Part model, mm, in its own coordinate system. A direction names the side the tool comes from. Give positions to 0.01 mm unless a question says otherwise; leave off trailing zeros. Loops run counter-clockwise (first coordinate to the right, second up) from the corner with the lowest first, then second, coordinate; pieces in that order, holes last. Notation, with made-up numbers: M 70.25,-33 L 76.25,-33 A14 cw 76.25,-22 Z; hole C -15.5,37 d7. An arc over 180 degrees is marked long. Put each result on its own line as item: value. Start each with the question number.
```python
from build123d import *

# Parameters (mm, degrees)
BOSS_EXTRUDE1_DEPTH = 3
SKETCH2_W           = 5
SKETCH2_H           = 5
BOSS_EXTRUDE2_DEPTH = 3
SKETCH3_W           = 5
SKETCH3_H           = 5
BOSS_EXTRUDE4_DEPTH = 3
SKETCH4_R           = 1.5
CUT_EXTRUDE1_DEPTH  = 27.537709019
CHAMFER1_SIZE       = 7
CHAMFER1_SIZE2      = 4.901452767
CHAMFER2_SIZE       = 7
CHAMFER2_SIZE2      = 4.901452767
SKETCH6_W           = 11
SKETCH6_H           = 3.5
BOSS_EXTRUDE5_DEPTH = 4.5
SKETCH9_W           = 11
SKETCH9_H           = 3.5
BOSS_EXTRUDE6_DEPTH = 3
FILLET1_R           = 5.5
FILLET2_R           = 3
SKETCH16_R          = 1.5
CUT_EXTRUDE7_DEPTH  = 30.857997254
SKETCH17_R          = 3.05
CUT_EXTRUDE8_DEPTH  = 2
SKETCH18_W          = 3
SKETCH18_H          = 8
BOSS_EXTRUDE7_DEPTH = 1
SKETCH19_W          = 3
SKETCH19_H          = 8
BOSS_EXTRUDE8_DEPTH = 1


# Some blends are built 0.0001 mm under size
with BuildPart() as part:
    # Sketch1 → Boss-Extrude1 (new body)
    with BuildSketch(Plane(origin=(0, 0, 0), x_dir=(1, 0, 0), z_dir=(0, 1, 0))):
        Polygon((-7.5, -12.5), (-7.5, 2.962729178), (0, 8.214285714), (7.5, 2.962729178), (7.5, -12.5), (12.5, -12.5), (12.5, 12.5), (-12.5, 12.5), (-12.5, -12.5), align=None)
    extrude(amount=BOSS_EXTRUDE1_DEPTH)

    # Sketch2 → Boss-Extrude2 (add)
    with BuildSketch(Plane.XY.offset(12.5)):
        with Locations((-10, 5.5)):
            Rectangle(SKETCH2_W, SKETCH2_H)
    extrude(amount=-BOSS_EXTRUDE2_DEPTH)

    # Sketch3 → Boss-Extrude4 (add)
    with BuildSketch(Plane.XY.offset(12.5)):
        with Locations((10, 5.5)):
            Rectangle(SKETCH3_W, SKETCH3_H)
    extrude(amount=-BOSS_EXTRUDE4_DEPTH)

    # Sketch4 → Cut-Extrude1 (cut, through all)
    with BuildSketch(Plane(origin=(0, 0, 9.5), x_dir=(-1, 0, 0), z_dir=(0, 0, -1))):
        with Locations((10, 5.5)):
            Circle(SKETCH4_R)
        with Locations(Location((-10, 5.5, 0), (0, 0, 180))):
            Circle(SKETCH4_R)
    extrude(amount=-CUT_EXTRUDE1_DEPTH, mode=Mode.SUBTRACT)

    # Chamfer1
    chamfer1_edges = [part.edges().sort_by_distance(p)[0] for p in [
        (-12.5, 1.5, -12.5),
    ]]
    chamfer1_side = [part.faces().sort_by_distance(p)[0] for p in [
        (0, 1.5, -12.5),
    ]]
    chamfer(chamfer1_edges, length=CHAMFER1_SIZE, length2=CHAMFER1_SIZE2, reference=chamfer1_side[0])

    # Chamfer2
    chamfer2_edges = [part.edges().sort_by_distance(p)[0] for p in [
        (12.5, 1.5, -12.5),
    ]]
    chamfer2_side = [part.faces().sort_by_distance(p)[0] for p in [
        (3.5, 1.5, -12.5),
    ]]
    chamfer(chamfer2_edges, length=CHAMFER2_SIZE, length2=CHAMFER2_SIZE2, reference=chamfer2_side[0])

    # Sketch6 → Boss-Extrude5 (add)
    with BuildSketch(Plane(origin=(0, 3, 0), x_dir=(1, 0, 0), z_dir=(0, 1, 0))):
        with Locations((0, 10.75)):
            Rectangle(SKETCH6_W, SKETCH6_H)
    extrude(amount=BOSS_EXTRUDE5_DEPTH)

    # Sketch9 → Boss-Extrude6 (add)
    with BuildSketch(Plane(origin=(0, 7.5, 0), x_dir=(1, 0, 0), z_dir=(0, 1, 0))):
        with Locations((0, 10.75)):
            Rectangle(SKETCH9_W, SKETCH9_H)
    extrude(amount=BOSS_EXTRUDE6_DEPTH)

    # Fillet1
    fillet1_edges = [part.edges().sort_by_distance(p)[0] for p in [
        (5.5, 10.5, -10.75),
        (-5.5, 10.5, -10.75),
    ]]
    fillet(fillet1_edges, radius=FILLET1_R - 0.0001)  # a hair under: the kernel refuses the full size

    # Fillet2
    # the kernel refuses this fillet: 3 mm, written as the material it adds along each edge
    with BuildSketch(Plane(origin=(-5.5, 3, -9), x_dir=(-1, 0, 0), z_dir=(0, 0, -1))) as fillet2_piece_1_section:
        with BuildLine():
            CenterArc((2.940982655, 3), FILLET2_R, 186.755728099, 83.244271901)
            Line((-0.038187449, 2.647089966), (-0.336104459, 2.611798962))
            ThreePointArc((-0.336104459, 2.611798962), (-0.3, 2.0001), (-0.3, 0))
            Line((-0.3, 0), (0, -0.3))
            Line((0, -0.3), (2.940982655, -0.3))
            Line((2.940982655, -0.3), (2.940982655, 0))
        make_face()
    fillet2_piece_1 = extrude(amount=3.5, mode=Mode.PRIVATE)
    fillet2_piece_1 = split(fillet2_piece_1, bisect_by=Plane(origin=(-8.304245999, 3.032166693, -10.536445813), z_dir=(0.5735764363510474, 0, 0.8191520442889909)), keep=Keep.TOP, mode=Mode.PRIVATE)
    add(fillet2_piece_1)
    with BuildSketch(Plane(origin=(5.5, 3, -12.5), x_dir=(-0.014424698824614252, 0.9998959586196051, 0), z_dir=(0, 0, 1))) as fillet2_piece_2_section:
        with BuildLine():
            CenterArc((2.957265087, -2.983950768), FILLET2_R, 95.929225072, 83.244271901)
            Line((-0.042422789, -2.940676671), (-0.342391577, -2.936349262))
            Line((-0.342391577, -2.936349262), (-0.299968788, 0.00432741))
            Line((-0.299968788, 0.00432741), (0.00432741, 0.299968788))
            ThreePointArc((0.00432741, 0.299968788), (2.004219316, 0.271117947), (2.616375433, 0.298395077))
            Line((2.616375433, 0.298395077), (2.647365401, 0))
        make_face()
    fillet2_piece_2 = extrude(amount=3.5, mode=Mode.PRIVATE)
    fillet2_piece_2 = split(fillet2_piece_2, bisect_by=Plane(origin=(6.733396297, 4.098580715, -11.636366615), z_dir=(-0.5735764363510474, 0, 0.8191520442889909)), keep=Keep.TOP, mode=Mode.PRIVATE)
    add(fillet2_piece_2)

    # Sketch16 → Cut-Extrude7 (cut, through all)
    with BuildSketch(Plane(origin=(0, 0, -12.5), x_dir=(-1, 0, 0), z_dir=(0, 0, -1))):
        with Locations((0, 6.5)):
            Circle(SKETCH16_R)
    extrude(amount=-CUT_EXTRUDE7_DEPTH, mode=Mode.SUBTRACT)

    # Sketch17 → Cut-Extrude8 (cut)
    with BuildSketch(Plane.XY.offset(-9)):
        with Locations((0, 6.5)):
            Circle(SKETCH17_R)
    extrude(amount=-CUT_EXTRUDE8_DEPTH, mode=Mode.SUBTRACT)

    # Sketch18 → Boss-Extrude7 (add)
    with BuildSketch(Plane.ZY.offset(-7.5)):
        with Locations((11, 4)):
            Rectangle(SKETCH18_W, SKETCH18_H)
    extrude(amount=BOSS_EXTRUDE7_DEPTH)

    # Sketch19 → Boss-Extrude8 (add)
    with BuildSketch(Plane(origin=(-7.5, 0, 0), x_dir=(0, 0, -1), z_dir=(1, 0, 0))):
        with Locations((-11, 4)):
            Rectangle(SKETCH19_W, SKETCH19_H)
    extrude(amount=BOSS_EXTRUDE8_DEPTH)


solid = part.part
```
1) Mould opens along X. For faces 5 (the flat face through (12.5, 2, 5)), 6 (the flat face through (0, 4, -12.5)), 7 (the cylindrical face through (-8.5, 5.57, 10.98)) say: +X half, -X half, draft (parallel to the pull), parting line (faces both ways), or undercut.
2) Band-saw the part on C-C on y = 7.5. Give the cut face in (x, z).
3) Which spindle directions (+Z, -Z, +X, -X, +Y, -Y) get a long thin tool onto all of the face, cutting with end or side? Do faces 1 (the cylindrical face through (6.095, 4.131, -10.386)), 2 (the flat face through (7.5, 1, 3)), 3 (the flat face through (-6.5, 4, 11)), 4 (the flat face through (1, 8, -11)). Say none if no direction does.
4) Band-saw the part on D-D on y = 4.5. Give the cut face in (x, z).
5) Wall check: L1, parallel to Y at x = 0, z = -10.4; L2, parallel to Z at x = -2.25, y = 7.75; L3, parallel to Z at x = 10.5, y = 7. Give the ranges that are in metal, low to high.
6) Band-saw the part on A-A on z = 11. Give the cut face in (x, y), then the cut area to 3 significant figures.
7) Band-saw the part on B-B on z = -2. Give the cut face in (x, y), then the cut area to 3 significant figures.
8) Pin check, flat tips, straight feed: pin 1 Ø3 at (x, y) = (-10, 5) entering from -Z; pin 2 Ø6 at (x, y) = (-1, 2.5) entering from +Z; pin 3 Ø6 at (x, y) = (-9, 4) entering from -Z; pin 4 Ø1.5 at (y, z) = (4, 0) entering from +X. Stop position of each tip, or through.
Evaluation:
1. face 5: +X half
1. face 6: draft
1. face 7: undercut
2. outline: M -12.5,9.5 L -6.5,9.5 L -6.5,12.5 L -12.5,12.5 Z; M -4.9,-12.5 L -1.12,-12.5 L -1.12,-11 L -2.88,-11 L -2.88,-9 L -4.9,-9 Z; M 1.12,-12.5 L 4.9,-12.5 L 4.9,-9 L 2.88,-9 L 2.88,-11 L 1.12,-11 Z; M 6.5,9.5 L 12.5,9.5 L 12.5,12.5 L 6.5,12.5 Z
3. face 1: -Z, +X, +Y
3. face 2: +Y, -Y
3. face 3: +Z, +Y, -Y
3. face 4: +Z
4. outline: M -12.5,9.5 L -11.12,9.5 L -11.12,12.5 L -12.5,12.5 Z; M -8.88,9.5 L -6.5,9.5 L -6.5,12.5 L -8.88,12.5 Z; M -5.84,-12.26 L -5.5,-12.5 L 5.5,-12.5 L 5.84,-12.26 L 5.84,-9 L 2.3,-9 L 2.3,-11 L -2.3,-11 L -2.3,-9 L -5.84,-9 Z; M 6.5,9.5 L 8.88,9.5 L 8.88,12.5 L 6.5,12.5 Z; M 11.12,9.5 L 12.5,9.5 L 12.5,12.5 L 11.12,12.5 Z
5. L1: 0 to 3.45, 9.55 to 10.5
5. L2: -12.5 to -11
5. L3: 9.5 to 12.5
6. outline: M -12.5,0 L -6.5,0 L -6.5,8 L -12.5,8 Z; M 6.5,0 L 12.5,0 L 12.5,8 L 6.5,8 Z; hole C -10,5.5 d3; hole C 10,5.5 d3
6. area: 81.9 mm2
7. outline: M -12.5,0 L -7.5,0 L -7.5,3 L -12.5,3 Z; M 7.5,0 L 12.5,0 L 12.5,3 L 7.5,3 Z
7. area: 30.0 mm2
8. pin 1: z = 9.5
8. pin 2: z = -5.41
8. pin 3: z = -12.15
8. pin 4: through
